Could you check a few things on this model? Use its own coordinates, in mm. A direction names the side the tool comes from. Coordinates: 2 decimals unless noted, no trailing zeros. Write each loop counter-clockwise with the first axis right and the second up, starting at its lowest first coordinate (ties: lowest second). Pieces come first, ordered by that corner, then holes. Notation, with made-up numbers: (13, 24.5) - (43, 24.5) arc R24 cw to (43, 49.5) - close; hole circle Ø6 at (12.5, 39.5). An arc over 180 degrees is marked (long way). Write item = value, one per line. Start each with the question number.
Autodesk Inventor part; units mm, degrees
ref_plane "YZ Plane" through (0, 0, 0) normal (1, 0, 0) x (0, 1, 0)
ref_plane "XZ Plane" through (0, 0, 0) normal (0, 1, 0) x (-1, 0, 0)
ref_plane "XY Plane" through (0, 0, 0) normal (0, 0, 1) x (1, 0, 0)
sketch "Sketch1" plane through (0, 0, 0) normal (0, 1, 0) x (-1, 0, 0)
  line L0 (0, 0) -> (0, -25.4)
  line L1 (0, -25.4) -> (3.175, -25.4)
  line L2 (3.175, -25.4) -> (3.175, -3.175)
  line L3 (3.175, -3.175) -> (6.35, -3.175)
  arc A0 (6.35, -3.175) -> (0, 0) centre (0.8204, -6.2968) ccw
  dimension "d0" = 25.4
  dimension "d1" = 3.175
  dimension "d2" = 22.225
  dimension "d3" = 3.175
  dimension "d4" = 6.35
revolve "Revolution1" add sketch "Sketch1" angle 360 about axis through (0, 0, 0) along (0, 0, -1)
sketch "Sketch2" plane through (0, 0, -25.4) normal (0, 0, -1) x (-1, 0, 0)
  line L0 (-1.5875, 0.9165) -> (0, 1.8331)
  line L1 (0, 1.8331) -> (1.5875, 0.9165)
  line L2 (1.5875, 0.9165) -> (1.5875, -0.9165)
  line L3 (1.5875, -0.9165) -> (0, -1.8331)
  line L4 (0, -1.8331) -> (-1.5875, -0.9165)
  line L5 (-1.5875, -0.9165) -> (-1.5875, 0.9165)
  point P0 (0, 0)
  point P1 (0, 0)
  dimension "d7" = 3.175
extrude "Extrusion1" cut sketch "Sketch2" against normal blind 31.75
sketch "Sketch3" plane through (0, 0, -25.4) normal (0, 0, -1) x (-1, 0, 0)
  line L0 (-1.5875, 0.9165) -> (0, 1.8331)
  line L1 (0, 1.8331) -> (1.5875, 0.9165)
  line L2 (1.5875, 0.9165) -> (1.5875, -0.9165)
  line L3 (1.5875, -0.9165) -> (0, -1.8331)
  line L4 (0, -1.8331) -> (-1.5875, -0.9165)
  line L5 (-1.5875, -0.9165) -> (-1.5875, 0.9165)
  point P0 (0, 0)
extrude "Extrusion2" add sketch "Sketch3" against normal blind 22.225
properties part number "14-20Bolt" material "Steel, Galvanized"
1) Which directions (+Z, -Z, +X, -X, +Y, -Y) give clear straight access to the entire face, cutting with the end or side of a thin tool? Please do faces 5 (the flat face through (0.783, -1.381, -1.606)), 6 (the flat face through (0, 0, -25.4)).
2) For P1, Ø0.9, axis at y = 0, z = -2, coming from the +X side; P2, Ø3, axis at y = -3.5, z = -21.5, coming from the -X side; P3, Ø3, axis at x = -3.5, z = -16.5, coming from the +Y side, each with a flat end and sliding along its axis, tell me the tip position at first contact or that it passes through.
3) Thinking about a two-plate mould opening in X: for faces 1 (the flat face through (1.588, 0, -2)), 2 (the flat face through (0.8, 1.37, -1.61)), 3 (the cylindrical face through (0.69, 3.1, -14.13)), 4 (the flat face through (2, 3, -3.175)), which applies, +X half, -X half, draft (parallel to the pull), parting line (faces both ways), or undercut?
4) Suppose I cut it at A-A on z = -23.5. Please give me the cut outline in (x, y) (3 decimals).
5) If I drill on probe 1 along X at (y, z) = (-2.75, -18); probe 2 along X at (y, z) = (-0.5, -21.5); probe 3 along Z at (x, y) = (-0.25, -5) (3 decimals), over which ranges is the centre line in solid material (lowest first)? Write a range as [from, to].
Reply:
q1.face_5 = +Z
q1.face_6 = -Z, +X, -X, +Y, -Y
q2.P1 = 5.87
q2.P2 = -2.47
q2.P3 = 2.47
q3.face_1 = undercut
q3.face_2 = undercut
q3.face_3 = parting line
q3.face_4 = draft
q4.outline = circle Ø6.35 at (0, 0)
q5.probe_1 = [-1.59, 1.59]
q5.probe_2 = [-3.14, 3.14]
q5.probe_3 = [-3.175, -1.522]
